Verification items for this drawing (mm, ordinates from the low corner). Round coordinates to 2 decimals unless told otherwise and drop trailing zeros. Loops run counter-clockwise (first coordinate to the right, second up) from the corner with the lowest first, then second, coordinate; pieces in that order, holes last. Notation, with made-up numbers: M -40,85 L -19,85 A28 cw -19,120 Z; hole C -22.5,36.5 d7. An arc over 180 degrees is marked long. Write item = value, one per line. Start each with the question number.
(1) Go/stop test with flat-tipped pins: P1, Ø12, axis at x = 10.5, z = 16.5, coming from the -Y side; P2, Ø7.5, axis at x = 26.5, z = 26.5, coming from the -Y side; P3, Ø2, axis at x = 31, z = 28, coming from the +Y side; P4, Ø0.7, axis at x = 30, y = 6.5, coming from the +Z side. Record where each tip stops, or that it passes through.
(2) Cross-section at B-B on x = 26.5. Record the boundary of the cut face in (y, z).
(3) Cross-section at C-C on y = 1. Record the boundary of the cut face in (x, z) (1 decimal), plus the area to 3 significant figures.
(4) Cross-section at A-A on z = 26.5. Record the boundary of the cut face in (x, y), plus the area to 3 significant figures.
(5) Scan lines: L1, parallel to Z at x = 26.5, y = 5.95; L2, parallel to Y at x = 19, z = 6; L3, parallel to Z at x = 17, y = 3.75. Record each from-to range of solid material in increasing order. Write a range as from..to.
(6) Mould release check, pull along X, two halves, no side actions. Record for the marked faces 1, 2, 3 and 4: pulls with the +X half, pulls with the -X half, needs draft (parallel to the pull), parting line crosses it, or undercut.
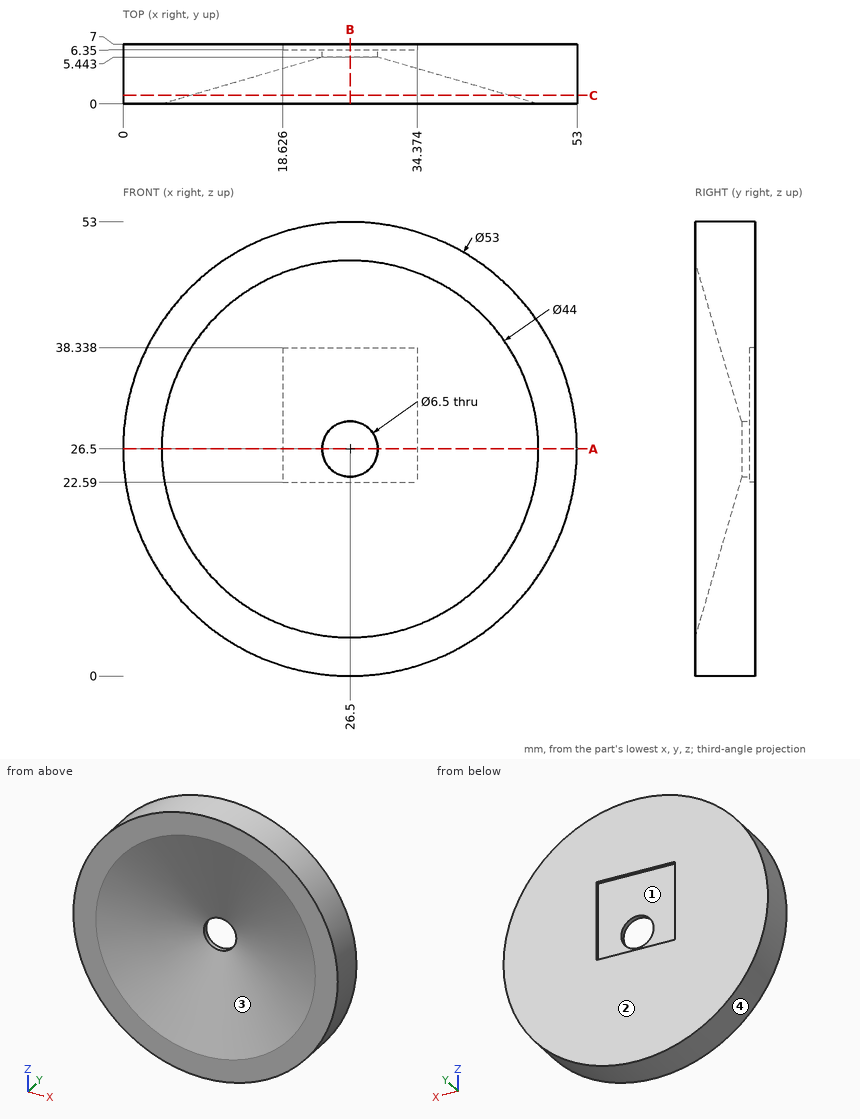
Result:
q1.P1 = 0
q1.P2 = 5.3
q1.P3 = 6.35
q1.P4 = 52.81
q2.outline = M 0,0 L 7,0 L 7,22.59 L 6.35,22.59 L 6.35,23.25 L 5.44,23.25 L 0,4.5 Z; M 0,48.5 L 5.44,29.75 L 6.35,29.75 L 6.35,38.34 L 7,38.34 L 7,53 L 0,53 Z
q3.outline = C 26.5,26.5 d53; hole C 26.5,26.5 d37.1
q3.area = 1,120 mm^2
q4.outline = M 0,0 L 4.5,0 L 23.25,5.44 L 23.25,6.35 L 18.63,6.35 L 18.63,7 L 0,7 Z; M 29.75,5.44 L 48.5,0 L 53,0 L 53,7 L 34.37,7 L 34.37,6.35 L 29.75,6.35 Z
q4.area = 217 mm^2
q5.L1 = 0..23.25, 29.75..53
q5.L2 = 0.05..7
q5.L3 = 1.76..51.24
q6.face_1 = undercut
q6.face_2 = needs draft
q6.face_3 = undercut
q6.face_4 = parting line crosses it
